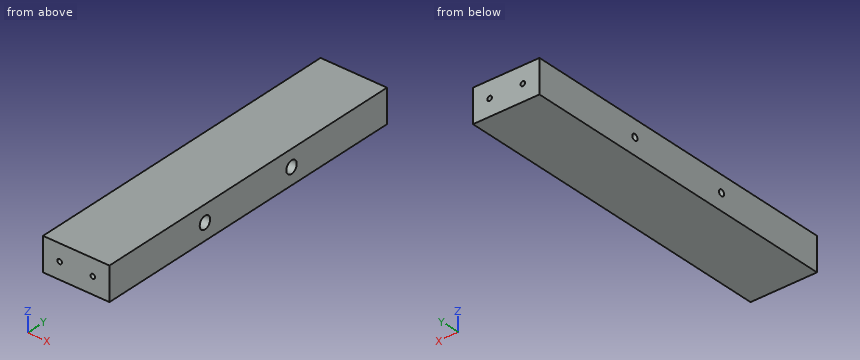
from build123d import *

# Parameters (mm, degrees)
SKETCH2_W                 = 25.4
SKETCH2_H                 = 127
BOSS_EXTRUDE1_DEPTH       = 6.35
SKETCH3_R                 = 1.190625
CUT_EXTRUDE2_DEPTH        = 26.4
SKETCH3_4_R               = 2.38125
SKETCH3_4_R_2             = 1.190625
CUT_EXTRUDE3_DEPTH        = 9.525
F_2_56_TAPPED_HOLE1_D     = 1.778
F_2_56_TAPPED_HOLE1_DEPTH = 10.668
F_2_56_TAPPED_HOLE1_TIP   = 0.53416509
F_2_56_TAPPED_HOLE2_D     = 1.778
F_2_56_TAPPED_HOLE2_DEPTH = 10.668
F_2_56_TAPPED_HOLE2_TIP   = 0.53416509


with BuildPart() as part:
    # Sketch2 → Boss-Extrude1 (new body, symmetric)
    with BuildSketch(Plane.XY):
        Rectangle(SKETCH2_W, SKETCH2_H)
    extrude(amount=BOSS_EXTRUDE1_DEPTH, both=True)

    # Sketch3 → Cut-Extrude2 (cut, through all)
    with BuildSketch(Plane(origin=(12.7, 0, 0), x_dir=(0, 0, -1), z_dir=(1, 0, 0))):
        with Locations((0, 19.812)):
            Circle(SKETCH3_R)
        with Locations((0, -19.812)):
            Circle(SKETCH3_R)
    extrude(amount=-CUT_EXTRUDE2_DEPTH, mode=Mode.SUBTRACT)

    # Sketch3_4 → Cut-Extrude3 (cut)
    with BuildSketch(Plane(origin=(12.7, 0, 0), x_dir=(0, 0, -1), z_dir=(1, 0, 0))):
        with Locations((0, 19.812)):
            Circle(SKETCH3_4_R)
        with Locations((0, 19.812)):
            Circle(SKETCH3_4_R_2, mode=Mode.SUBTRACT)
        with Locations((0, -19.812)):
            Circle(SKETCH3_4_R)
        with Locations((0, -19.812)):
            Circle(SKETCH3_4_R_2, mode=Mode.SUBTRACT)
    extrude(amount=-CUT_EXTRUDE3_DEPTH, mode=Mode.SUBTRACT)

    # 2-56 Tapped Hole1
    with Locations(Plane(origin=(0, 63.5, 0), x_dir=(-1, 0, 0), z_dir=(0, 1, 0))):
        with Locations((6.35, 0), (-6.35, 0)):
            Hole(F_2_56_TAPPED_HOLE1_D / 2, depth=F_2_56_TAPPED_HOLE1_DEPTH)
            with Locations((0, 0, -(F_2_56_TAPPED_HOLE1_DEPTH + F_2_56_TAPPED_HOLE1_TIP / 2))):  # 118° drill point
                Cone(0, F_2_56_TAPPED_HOLE1_D / 2, F_2_56_TAPPED_HOLE1_TIP, mode=Mode.SUBTRACT)

    # 2-56 Tapped Hole2
    with Locations(Plane.XZ.offset(63.5)):
        with Locations((6.35, 0), (-6.35, 0)):
            Hole(F_2_56_TAPPED_HOLE2_D / 2, depth=F_2_56_TAPPED_HOLE2_DEPTH)
            with Locations((0, 0, -(F_2_56_TAPPED_HOLE2_DEPTH + F_2_56_TAPPED_HOLE2_TIP / 2))):  # 118° drill point
                Cone(0, F_2_56_TAPPED_HOLE2_D / 2, F_2_56_TAPPED_HOLE2_TIP, mode=Mode.SUBTRACT)


solid = part.part
Design review of the part built by this model. Coordinates are the model's own, in mm. Coordinates: 2 decimals unless noted, no trailing zeros. Write each loop counter-clockwise with the first axis right and the second up, starting at its lowest first coordinate (ties: lowest second). Pieces come first, ordered by that corner, then holes. Notation, with made-up numbers: (36, -16) - (87, -16) arc R35 ccw to (87, 17) - close; hole circle Ø7 at (70.5, 84.5). An arc over 180 degrees is marked (long way). Use one line per item in the form item = value.
Q1. For probe 1 along Y at (x, z) = (-4.25, 0); probe 2 along X at (y, z) = (57.25, 0); probe 3 along Y at (x, z) = (6.5, 0), list the stretches that pass through material, from the lowest coordinate up.
Taken from the geometry:
probe_1 = -63.5 to -21, -18.62 to 18.62, 21 to 63.5
probe_2 = -12.7 to -7.24, -5.46 to 5.46, 7.24 to 12.7
probe_3 = -52.39 to -22.19, -17.43 to 17.43, 22.19 to 52.39
Q2. Consider section A-A (x = 11.25). Write out the cut boundary in (y, z), plus the area to 3 significant figures.
Taken from the geometry:
outline = (-63.5, -6.35) - (63.5, -6.35) - (63.5, 6.35) - (-63.5, 6.35) - close; hole circle Ø4.76 at (-19.81, 0); hole circle Ø4.76 at (19.81, 0)
area = 1,580 mm^2
Q3. Insertion check: pin 1 Ø1.1 at (x, z) = (-6.35, 0) entering from +Y; pin 2 Ø1.6 at (x, z) = (-6.35, 0) entering from -Y; pin 3 Ø1.9 at (y, z) = (19.812, 0) entering from -X; pin 4 Ø1.1 at (x, z) = (6.35, 0) entering from -Y. Each pin has a flat end and moves straight along its axis. Give the tip position at first contact, or say it passes through.
Taken from the geometry:
pin_1 = 52.63
pin_2 = -52.78
pin_3 = through
pin_4 = -52.63
